Here's how the part is built. I have some questions about the finished solid (model axes, mm). Face numbers are marked on the shaded views. Give positions to 0.01 mm unless a question says otherwise; leave off trailing zeros. Return JSON: item names as keys, results as strings. Group by question number.
(1) If we section it at A-A (z = 0): State how many separate pieces and enclosed holes the cut face has, then the cut area to 3 significant figures.
(2) If we mould it in two halves opening along Y, with no side actions, what happens to the marked faces 1, 2, 3 and 4? For each: released by +Y, released by -Y, zero draft, split by the parting line, or undercut.
(3) I need wall thicknesses on probe 1 along X at (y, z) = (1.25, 0); probe 2 along Y at (x, z) = (-5, 19); probe 3 along Z at (x, y) = (17, 1.5). Which ranges of each line are inside material? Lowest first, please. Write a range as [from, to].
(4) For P1, Ø1, axis at y = 5.5, z = 4.5, coming from the -X side; P2, Ø2, axis at y = 4.5, z = 17, coming from the -X side; P3, Ø1.5, axis at y = 3.5, z = -9, coming from the -X side, each with a flat end and sliding along its axis, tell me the tip position at first contact or that it passes through.
```python
from build123d import *

# Parameters (mm, degrees)
EXTRUDE_1_DEPTH     = 8
SKETCH_2_R          = 22
EXTRUDE_2_DEPTH     = 1
FILLET_1_R          = 0.5
EXTRUDE_START       = 1
SKETCH_3_R          = 22
EXTRUDE_3_DEPTH     = 1
FILLET_2_R          = 0.5
HOLE_WIZARD_M3_1_D  = 2.5
SKETCH_9_R          = 9
CUT_EXTRUDE_2_DEPTH = 33.680269442


with BuildPart() as part:
    # 草图1 → 凸台-拉伸1 (new body)
    with BuildSketch(Plane(origin=(0, 0, 0), x_dir=(1, 0, 0), z_dir=(0, 1, 0))):
        with BuildLine():
            ThreePointArc((-19.598458084, 3.987535674), (-19.753766812, 3.128689301), (-19.871457558, 2.263884825))
            ThreePointArc((-19.871457558, 2.263884825), (-19.739336252, 1.865206806), (-19.349906932, 1.707901346))
            ThreePointArc((-19.349906932, 1.707901346), (-17.555213412, 0), (-19.349906932, -1.707901346))
            ThreePointArc((-19.349906932, -1.707901346), (-19.739336252, -1.865206806), (-19.871457558, -2.263884825))
            ThreePointArc((-19.871457558, -2.263884825), (-19.753766812, -3.128689301), (-19.598458084, -3.987535674))
            ThreePointArc((-19.598458084, -3.987535674), (-19.349604971, -4.325873273), (-18.930625618, -4.355139377))
            ThreePointArc((-18.930625618, -4.355139377), (-16.69600011, -5.424859284), (-17.875084537, -7.603760786))
            ThreePointArc((-17.875084537, -7.603760786), (-18.196843769, -7.873707446), (-18.199300315, -8.293700504))
            ThreePointArc((-18.199300315, -8.293700504), (-17.820130484, -9.079809995), (-17.407024981, -9.848628398))
            ThreePointArc((-17.407024981, -9.848628398), (-17.065799538, -10.093506735), (-16.658282771, -9.991868714))
            ThreePointArc((-16.658282771, -9.991868714), (-14.20246599, -10.318695544), (-14.650524324, -12.755311142))
            ThreePointArc((-14.650524324, -12.755311142), (-14.873117433, -13.111474743), (-14.745668755, -13.511670991))
            ThreePointArc((-14.745668755, -13.511670991), (-14.142135624, -14.142135624), (-13.511670991, -14.745668755))
            ThreePointArc((-13.511670991, -14.745668755), (-13.111474743, -14.873117433), (-12.755311142, -14.650524324))
            ThreePointArc((-12.755311142, -14.650524324), (-10.318695544, -14.20246599), (-9.991868714, -16.658282771))
            ThreePointArc((-9.991868714, -16.658282771), (-10.093506735, -17.065799538), (-9.848628398, -17.407024981))
            ThreePointArc((-9.848628398, -17.407024981), (-9.079809995, -17.820130484), (-8.293700504, -18.199300315))
            ThreePointArc((-8.293700504, -18.199300315), (-7.873707446, -18.196843769), (-7.603760786, -17.875084537))
            ThreePointArc((-7.603760786, -17.875084537), (-5.424859284, -16.69600011), (-4.355139377, -18.930625618))
            ThreePointArc((-4.355139377, -18.930625618), (-4.325873273, -19.349604971), (-3.987535674, -19.598458084))
            ThreePointArc((-3.987535674, -19.598458084), (-3.128689301, -19.753766812), (-2.263884825, -19.871457558))
            ThreePointArc((-2.263884825, -19.871457558), (-1.865206806, -19.739336252), (-1.707901346, -19.349906932))
            ThreePointArc((-1.707901346, -19.349906932), (0, -17.555213412), (1.707901346, -19.349906932))
            ThreePointArc((1.707901346, -19.349906932), (1.865206806, -19.739336252), (2.263884825, -19.871457558))
            ThreePointArc((2.263884825, -19.871457558), (3.128689301, -19.753766812), (3.987535674, -19.598458084))
            ThreePointArc((3.987535674, -19.598458084), (4.325873273, -19.349604971), (4.355139377, -18.930625618))
            ThreePointArc((4.355139377, -18.930625618), (5.424859284, -16.69600011), (7.603760786, -17.875084537))
            ThreePointArc((7.603760786, -17.875084537), (7.873707446, -18.196843769), (8.293700504, -18.199300315))
            ThreePointArc((8.293700504, -18.199300315), (9.079809995, -17.820130484), (9.848628398, -17.407024981))
            ThreePointArc((9.848628398, -17.407024981), (10.093506735, -17.065799538), (9.991868714, -16.658282771))
            ThreePointArc((9.991868714, -16.658282771), (10.318695544, -14.20246599), (12.755311142, -14.650524324))
            ThreePointArc((12.755311142, -14.650524324), (13.111474743, -14.873117433), (13.511670991, -14.745668755))
            ThreePointArc((13.511670991, -14.745668755), (14.142135624, -14.142135624), (14.745668755, -13.511670991))
            ThreePointArc((14.745668755, -13.511670991), (14.873117433, -13.111474743), (14.650524324, -12.755311142))
            ThreePointArc((14.650524324, -12.755311142), (14.20246599, -10.318695544), (16.658282771, -9.991868714))
            ThreePointArc((16.658282771, -9.991868714), (17.065799538, -10.093506735), (17.407024981, -9.848628398))
            ThreePointArc((17.407024981, -9.848628398), (17.820130484, -9.079809995), (18.199300315, -8.293700504))
            ThreePointArc((18.199300315, -8.293700504), (18.196843769, -7.873707446), (17.875084537, -7.603760786))
            ThreePointArc((17.875084537, -7.603760786), (16.69600011, -5.424859284), (18.930625618, -4.355139377))
            ThreePointArc((18.930625618, -4.355139377), (19.349604971, -4.325873273), (19.598458084, -3.987535674))
            ThreePointArc((19.598458084, -3.987535674), (19.753766812, -3.128689301), (19.871457558, -2.263884825))
            ThreePointArc((19.871457558, -2.263884825), (19.739336252, -1.865206806), (19.349906932, -1.707901346))
            ThreePointArc((19.349906932, -1.707901346), (17.555213412, 0), (19.349906932, 1.707901346))
            ThreePointArc((19.349906932, 1.707901346), (19.739336252, 1.865206806), (19.871457558, 2.263884825))
            ThreePointArc((19.871457558, 2.263884825), (19.753766812, 3.128689301), (19.598458084, 3.987535674))
            ThreePointArc((19.598458084, 3.987535674), (19.349604971, 4.325873273), (18.930625618, 4.355139377))
            ThreePointArc((18.930625618, 4.355139377), (16.69600011, 5.424859284), (17.875084537, 7.603760786))
            ThreePointArc((17.875084537, 7.603760786), (18.196843769, 7.873707446), (18.199300315, 8.293700504))
            ThreePointArc((18.199300315, 8.293700504), (17.820130484, 9.079809995), (17.407024981, 9.848628398))
            ThreePointArc((17.407024981, 9.848628398), (17.065799538, 10.093506735), (16.658282771, 9.991868714))
            ThreePointArc((16.658282771, 9.991868714), (14.20246599, 10.318695544), (14.650524324, 12.755311142))
            ThreePointArc((14.650524324, 12.755311142), (14.873117433, 13.111474743), (14.745668755, 13.511670991))
            ThreePointArc((14.745668755, 13.511670991), (14.142135624, 14.142135624), (13.511670991, 14.745668755))
            ThreePointArc((13.511670991, 14.745668755), (13.111474743, 14.873117433), (12.755311142, 14.650524324))
            ThreePointArc((12.755311142, 14.650524324), (10.318695544, 14.20246599), (9.991868714, 16.658282771))
            ThreePointArc((9.991868714, 16.658282771), (10.093506735, 17.065799538), (9.848628398, 17.407024981))
            ThreePointArc((9.848628398, 17.407024981), (9.079809995, 17.820130484), (8.293700504, 18.199300315))
            ThreePointArc((8.293700504, 18.199300315), (7.873707446, 18.196843769), (7.603760786, 17.875084537))
            ThreePointArc((7.603760786, 17.875084537), (5.424859284, 16.69600011), (4.355139377, 18.930625618))
            ThreePointArc((4.355139377, 18.930625618), (4.325873273, 19.349604971), (3.987535674, 19.598458084))
            ThreePointArc((3.987535674, 19.598458084), (3.128689301, 19.753766812), (2.263884825, 19.871457558))
            ThreePointArc((2.263884825, 19.871457558), (1.865206806, 19.739336252), (1.707901346, 19.349906932))
            ThreePointArc((1.707901346, 19.349906932), (0, 17.555213412), (-1.707901346, 19.349906932))
            ThreePointArc((-1.707901346, 19.349906932), (-1.865206806, 19.739336252), (-2.263884825, 19.871457558))
            ThreePointArc((-2.263884825, 19.871457558), (-3.128689301, 19.753766812), (-3.987535674, 19.598458084))
            ThreePointArc((-3.987535674, 19.598458084), (-4.325873273, 19.349604971), (-4.355139377, 18.930625618))
            ThreePointArc((-4.355139377, 18.930625618), (-5.424859284, 16.69600011), (-7.603760786, 17.875084537))
            ThreePointArc((-7.603760786, 17.875084537), (-7.873707446, 18.196843769), (-8.293700504, 18.199300315))
            ThreePointArc((-8.293700504, 18.199300315), (-9.079809995, 17.820130484), (-9.848628398, 17.407024981))
            ThreePointArc((-9.848628398, 17.407024981), (-10.093506735, 17.065799538), (-9.991868714, 16.658282771))
            ThreePointArc((-9.991868714, 16.658282771), (-10.318695544, 14.20246599), (-12.755311142, 14.650524324))
            ThreePointArc((-12.755311142, 14.650524324), (-13.111474743, 14.873117433), (-13.511670991, 14.745668755))
            ThreePointArc((-13.511670991, 14.745668755), (-14.142135624, 14.142135624), (-14.745668755, 13.511670991))
            ThreePointArc((-14.745668755, 13.511670991), (-14.873117433, 13.111474743), (-14.650524324, 12.755311142))
            ThreePointArc((-14.650524324, 12.755311142), (-14.20246599, 10.318695544), (-16.658282771, 9.991868714))
            ThreePointArc((-16.658282771, 9.991868714), (-17.065799538, 10.093506735), (-17.407024981, 9.848628398))
            ThreePointArc((-17.407024981, 9.848628398), (-17.820130484, 9.079809995), (-18.199300315, 8.293700504))
            ThreePointArc((-18.199300315, 8.293700504), (-18.196843769, 7.873707446), (-17.875084537, 7.603760786))
            ThreePointArc((-17.875084537, 7.603760786), (-16.69600011, 5.424859284), (-18.930625618, 4.355139377))
            ThreePointArc((-18.930625618, 4.355139377), (-19.349604971, 4.325873273), (-19.598458084, 3.987535674))
        make_face()
    extrude(amount=EXTRUDE_1_DEPTH)

    # 草图2 → 凸台-拉伸2 (add)
    with BuildSketch(Plane(origin=(0, 0, 0), x_dir=(1, 0, 0), z_dir=(0, 1, 0))):
        with Locations(Location((0, 0, 0), (0, 0, 270))):
            Circle(SKETCH_2_R)
    extrude(amount=-EXTRUDE_2_DEPTH)

    # 圆角1
    fillet_1_edges = [part.edges().sort_by_distance(p)[0] for p in [
        (0, 0, -22),
        (0, -1, -22),
    ]]
    fillet(fillet_1_edges, radius=FILLET_1_R - 0.0001)  # a hair under: the kernel refuses the full size

    # 草图3 → 凸台-拉伸3 (add)
    with BuildSketch(Plane(origin=(0, 8, 0), x_dir=(1, 0, 0), z_dir=(0, 1, 0)).offset(EXTRUDE_START)):
        with Locations(Location((0, 0, 0), (0, 0, 270))):
            Circle(SKETCH_3_R)
    extrude(amount=-EXTRUDE_3_DEPTH)

    # 圆角2
    fillet_2_edges = [part.edges().sort_by_distance(p)[0] for p in [
        (0, 8, -22),
        (0, 9, -22),
    ]]
    fillet(fillet_2_edges, radius=FILLET_2_R - 0.0001)  # a hair under: the kernel refuses the full size

    # M3 螺纹孔的螺纹孔钻头1 (through all)
    with Locations(Plane(origin=(-10.960155108, 9, -10.960155108), x_dir=(0, 0, 1), z_dir=(0, 1, 0))):
        with Locations((0, 0), (-4.539844892, 10.960155108), (0, 21.920310216), (10.960155108, 26.460155108), (21.920310216, 21.920310216), (26.460155108, 10.960155108), (21.920310216, 0), (10.960155108, -4.539844892)):
            Hole(HOLE_WIZARD_M3_1_D / 2)

    # 草图9 → 切除-拉伸2 (cut, through all)
    with BuildSketch(Plane(origin=(0, 9, 0), x_dir=(1, 0, 0), z_dir=(0, 1, 0))):
        with Locations(Location((0, 0, 0), (0, 0, 270))):
            Circle(SKETCH_9_R)
    extrude(amount=-CUT_EXTRUDE_2_DEPTH, mode=Mode.SUBTRACT)


solid = part.part
```
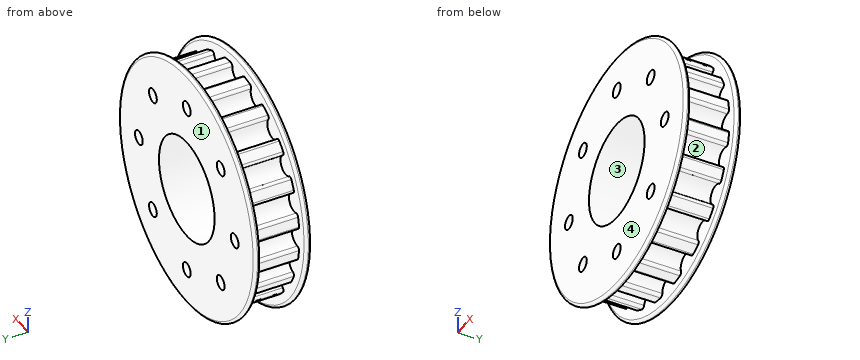
Values:
{
 "1": {"separate pieces": "4", "enclosed holes": "0", "area": "138 mm2"},
 "2": {"face 1": "released by +Y", "face 2": "undercut", "face 3": "zero draft", "face 4": "released by -Y"},
 "3": {"probe 1": "[-17.56, -16.75], [-14.25, -9], [9, 14.25], [16.75, 17.56]", "probe 2": "[-1, 0], [8, 9]", "probe 3": "[-10.1, -7.04], [-4.87, 4.87], [7.04, 10.1]"},
 "4": {"P1": "x = -19.6", "P2": "x = -10.1", "P3": "x = -18.22"}
}
